CAD build for the part. Positions are in the model's coordinates, mm. A direction names the side the tool comes from. Coordinates: 2 decimals unless noted, no trailing zeros. Order: outer loops, then holes, each group sorted by start corner. A loop starts at its lowest first (then second) coordinate and runs counter-clockwise, first axis right, second up. Notation, with made-up numbers: M 24.5,-8.5 L 59.5,-8.5 A15 ccw 59.5,20.5 Z; hole C 53,5 d4. An arc over 180 degrees is marked long. Write item = value, one per line. Start each with the question number.
```python
from build123d import *

# Parameters (mm, degrees)
BOSS_EXTRUDE2_DEPTH     = 6.35
CUT_EXTRUDE1_REACH      = 129.376
CUT_EXTRUDE2_DEPTH      = 128.37561853
CUT_EXTRUDE2_DEPTH_BACK = 128.37561853
SKETCH5_R               = 3.175
SKETCH6_R               = 1.984375
CUT_EXTRUDE3_DEPTH      = 128.37561853


with BuildPart() as part:
    # Sketch3 → Boss-Extrude2 (new body)
    with BuildSketch(Plane(origin=(0, 0, 0), x_dir=(0, 0, -1), z_dir=(1, 0, 0))):
        with BuildLine():
            Line((-57.15, -110.236), (57.15, -110.236))
            ThreePointArc((57.15, -110.236), (61.640128061, -108.376128061), (63.5, -103.886))
            Line((63.5, -103.886), (63.5, 103.886))
            ThreePointArc((63.5, 103.886), (61.640128061, 108.376128061), (57.15, 110.236))
            Line((57.15, 110.236), (-57.15, 110.236))
            ThreePointArc((-57.15, 110.236), (-61.640128061, 108.376128061), (-63.5, 103.886))
            Line((-63.5, 103.886), (-63.5, -103.886))
            ThreePointArc((-63.5, -103.886), (-61.640128061, -108.376128061), (-57.15, -110.236))
        make_face()
        with BuildLine():
            Line((-31.75, -67.564), (31.75, -67.564))
            ThreePointArc((31.75, -67.564), (36.240128061, -65.704128061), (38.1, -61.214))
            Line((38.1, -61.214), (38.1, 78.486))
            ThreePointArc((38.1, 78.486), (36.240128061, 82.976128061), (31.75, 84.836))
            Line((31.75, 84.836), (-31.75, 84.836))
            ThreePointArc((-31.75, 84.836), (-36.240128061, 82.976128061), (-38.1, 78.486))
            Line((-38.1, 78.486), (-38.1, -61.214))
            ThreePointArc((-38.1, -61.214), (-36.240128061, -65.704128061), (-31.75, -67.564))
        make_face(mode=Mode.SUBTRACT)
    extrude(amount=BOSS_EXTRUDE2_DEPTH)

    # Sketch4 → Cut-Extrude1 (cut, up to next)
    with BuildSketch(Plane(origin=(6.35, 0, 0), x_dir=(0, 0, -1), z_dir=(1, 0, 0)), mode=Mode.PRIVATE) as cut_extrude1_sk1:
        Polygon((0, -97.536), (-8.980256121, -88.555743879), (-9.878281733, -89.453769491), (0, -99.332051224), (9.878281733, -89.453769491), (8.980256121, -88.555743879), align=None)
    cut_extrude1_tool1 = extrude(cut_extrude1_sk1.sketch, amount=-CUT_EXTRUDE1_REACH, mode=Mode.PRIVATE) & part.part
    add(cut_extrude1_tool1.solids().sort_by_distance((6.35, -93.205002, 4.649259))[0], mode=Mode.SUBTRACT)

    # Sketch5 → Cut-Extrude2 (cut, two sides: drawn at the far end of the back side and taken through both)
    with BuildSketch(Plane(origin=(6.35, 0, 0), x_dir=(0, 0, -1), z_dir=(1, 0, 0)).offset(-CUT_EXTRUDE2_DEPTH_BACK)):
        with Locations((-31.75, 97.536)):
            Circle(SKETCH5_R)
        with Locations((31.75, 97.536)):
            Circle(SKETCH5_R)
    extrude(amount=CUT_EXTRUDE2_DEPTH + CUT_EXTRUDE2_DEPTH_BACK, mode=Mode.SUBTRACT)

    # Sketch6 → Cut-Extrude3 (cut, through all)
    with BuildSketch(Plane(origin=(6.35, 0, 0), x_dir=(0, 0, -1), z_dir=(1, 0, 0))):
        with Locations((-50.8, 34.036)):
            Circle(SKETCH6_R)
        with Locations(Location((50.8, 34.036, 0), (0, 0, 180))):
            Circle(SKETCH6_R)
    extrude(amount=-CUT_EXTRUDE3_DEPTH, mode=Mode.SUBTRACT)


solid = part.part
```
1. Flat gauge pin, fed straight in: pin 1 (2.5 mm diameter, centred on y = 34.036, z = -50.8, fed in from +X). Where does the tip first touch, or does it go through?
2. 3-axis set-ups, long thin cutter, end or side, ignore diameter. For faces 4 (the flat face through (3.219, -93.109, 4.427)), 5 (the cylindrical face through (3.131, -108.326, 61.689)): which of +Z, -Z, +X, -X, +Y, -Y reach the whole face in a straight line?
3. Slice it at A-A (y = 43). Write the cut outline in (x, z), plus the area to 3 significant figures.
4. Slice it at C-C (y = -95). Write the cut outline in (x, z), plus the area to 3 significant figures.
5. Probe L1, parallel to Y at x = 4.25, z = 31.75; L2, parallel to Z at x = 4, y = 22.5; L3, parallel to Y at x = 4, z = -50.8. List the from-to ranges inside material, lowest first.
6. Mould opens along Z. For faces 1 (the flat face through (3, -110.236, 1)), 2 (the cylindrical face through (3.131, 108.326, -61.689)), 3 (the cylindrical face through (3.131, 100.684, -31.337)) say: released by +Z, released by -Z, zero draft, split by the parting line, or undercut.
7. Slice it at D-D (x = 3). Write the cut outline in (y, z) (3 decimals).
8. Slice it at B-B (z = -18.5). Write the cut outline in (x, y).
Calculated:
q1.pin_1 = through
q2.face_4 = +X, -X
q2.face_5 = +Z, +X, -X, -Y
q3.outline = M 0,-63.5 L 6.35,-63.5 L 6.35,-38.1 L 0,-38.1 Z; M 0,38.1 L 6.35,38.1 L 6.35,63.5 L 0,63.5 Z
q3.area = 323 mm²
q4.outline = M 0,-63.5 L 6.35,-63.5 L 6.35,-4.33 L 0,-4.33 Z; M 0,-2.54 L 6.35,-2.54 L 6.35,2.54 L 0,2.54 Z; M 0,4.33 L 6.35,4.33 L 6.35,63.5 L 0,63.5 Z
q4.area = 784 mm²
q5.L1 = -110.24 to -67.56, 84.84 to 94.36, 100.71 to 110.24
q5.L2 = -63.5 to -38.1, 38.1 to 63.5
q5.L3 = -110.24 to 32.05, 36.02 to 110.24
q6.face_1 = zero draft
q6.face_2 = released by -Z
q6.face_3 = undercut
q7.outline = M -110.236,-57.15 A6.35 ccw -103.886,-63.5 L 103.886,-63.5 A6.35 ccw 110.236,-57.15 L 110.236,57.15 A6.35 ccw 103.886,63.5 L -103.886,63.5 A6.35 ccw -110.236,57.15 Z; hole M -99.332,0 L -89.454,-9.878 L -88.556,-8.98 L -97.536,0 L -88.556,8.98 L -89.454,9.878 Z; hole M -67.564,-31.75 A6.35 ccw -61.214,-38.1 L 78.486,-38.1 A6.35 ccw 84.836,-31.75 L 84.836,31.75 A6.35 ccw 78.486,38.1 L -61.214,38.1 A6.35 ccw -67.564,31.75 Z; hole C 34.036,-50.8 d3.969; hole C 34.036,50.8 d3.969; hole C 97.536,-31.75 d6.35; hole C 97.536,31.75 d6.35
q8.outline = M 0,-110.24 L 6.35,-110.24 L 6.35,-67.56 L 0,-67.56 Z; M 0,84.84 L 6.35,84.84 L 6.35,110.24 L 0,110.24 Z
